Design review of the part shown in the three views and the two pictorial views. Dimensions are in mm from the part's minimum x, y and z. A direction names the side the tool comes from. Coordinates: 2 decimals unless noted, no trailing zeros. Loops run counter-clockwise (first coordinate to the right, second up) from the corner with the lowest first, then second, coordinate; pieces in that order, holes last.
Q1. Add section A-A on x = 5. Give the boundary of the cut face in (y, z), and give its area (3 significant figures).
Q2. Machinability: for the marked faces 1, 2, 3 and 4, which of the approach directions +Z, -Z, +X, -X, +Y, -Y give a long, thin tool a straight path to every point of the face, cutting with its end or side? Answer none if there is none.
Q3. Wall thickness on probe 1 along Y at (x, z) = (9.5, 3.8); probe 2 along X at (y, z) = (2, 2); probe 3 along X at (y, z) = (4.5, 4.4): over which ranges is each line inside the solid? List them lowest first.
Q4. For P1, Ø1, axis at y = 6, z = 3.5, coming from the -X side; P2, Ø1, axis at y = 3.5, z = 2, coming from the +X side; P3, Ø2, axis at x = 7.5, z = 2.5, coming from the +Y side, all flat-tipped, find the tip position at first contact; note any pin that passes through.
Q5. Add section B-B on z = 3.5. Give the boundary of the cut face in (x, y).
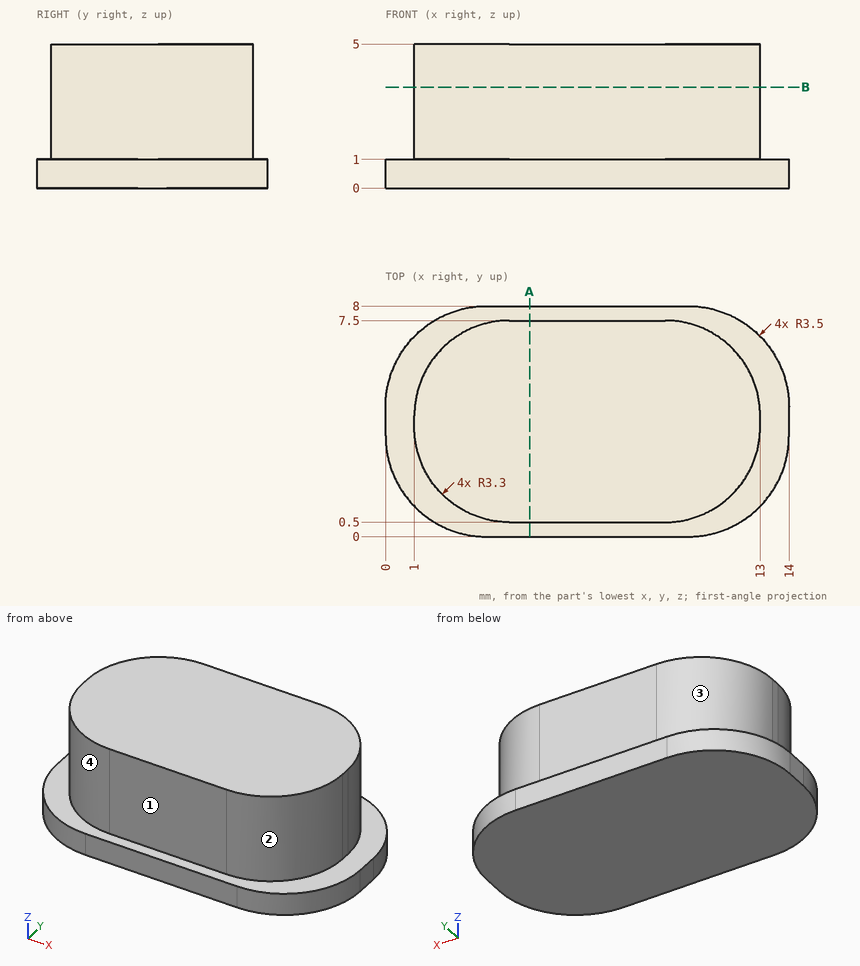
Entries:
1. outline: (0, 0) - (8, 0) - (8, 1) - (7.5, 1) - (7.5, 5) - (0.5, 5) - (0.5, 1) - (0, 1) - close
1. area: 36.0 mm2
2. face 1: +Z, +X, -X, -Y
2. face 2: +Z, +X, -Y
2. face 3: +Z, -X, +Y
2. face 4: +Z, -X, -Y
3. probe 1: y = 0.5 to 7.5
3. probe 2: x = 1.53 to 12.47
3. probe 3: x = 1.01 to 12.99
4. P1: stops at x = 1.27
4. P2: stops at x = 13
4. P3: stops at y = 7.5
5. outline: (1, 3.8) arc R3.3 ccw to (4.3, 0.5) - (9.7, 0.5) arc R3.3 ccw to (13, 3.8) - (13, 4.2) arc R3.3 ccw to (9.7, 7.5) - (4.3, 7.5) arc R3.3 ccw to (1, 4.2) - close
